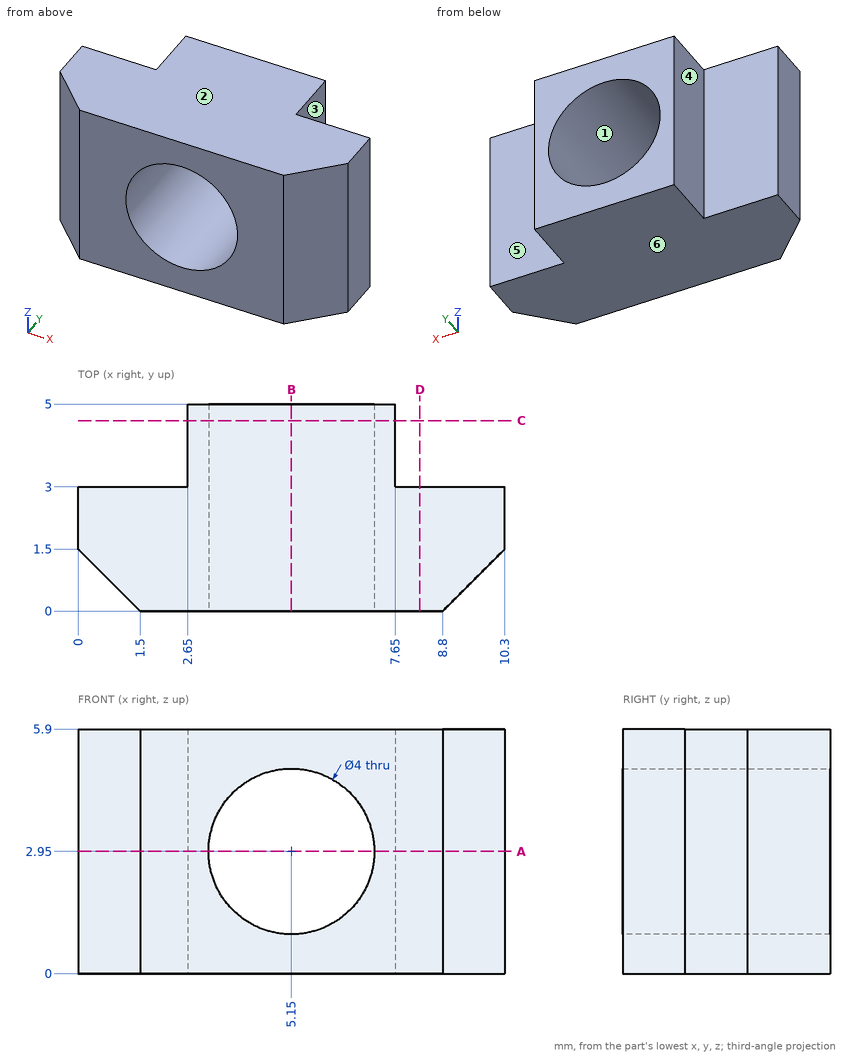
Source: three-view drawing plus pictorial views. Frame: mm from the lowest corner of the part. A direction names the side the tool comes from. Give positions to 0.01 mm unless a question says otherwise; leave off trailing zeros. Loops run counter-clockwise (first coordinate to the right, second up) from the corner with the lowest first, then second, coordinate; pieces in that order, holes last. Notation, with made-up numbers: M -16.75,12 L 3.25,12 A16 cw 3.25,22 Z; hole C 12,63 d1. An arc over 180 degrees is marked long. Use CSV: the item, a comma, the result in double quotes.
(1) Pull-direction query (X, two-part tool) for the marked faces 1, 2 and 3; classes: pulls with the +X half, pulls with the -X half, needs draft (parallel to the pull), parting line crosses it, or undercut.
Outcome:
face 1,"undercut"
face 2,"needs draft"
face 3,"pulls with the +X half"
(2) Set-up query: the marked faces 4, 5 and 6. Return all of +Z, -Z, +X, -X, +Y, -Y with unobstructed straight access to the full face (end or side cutting, diameter ignored); none if empty.
Outcome:
face 4,"+Z, -Z, -X, +Y"
face 5,"+Z, -Z, +X, +Y"
face 6,"-Z, +X, -X, +Y, -Y"
(3) Material intervals for L1, parallel to X at y = 3.75, z = 2.95; L2, parallel to X at y = 2, z = 2.95; L3, parallel to Y at x = 8.5, z = 4.3, sorted ascending. Write a range as [from, to].
Outcome:
L1,"x = [2.65, 3.15], [7.15, 7.65]"
L2,"x = [0, 3.15], [7.15, 10.3]"
L3,"y = [0, 3]"
(4) Section A-A, the plane z = 2.95. Return loops of the section in (x, y).
Outcome:
outline,"M 0,1.5 L 1.5,0 L 3.15,0 L 3.15,5 L 2.65,5 L 2.65,3 L 0,3 Z; M 7.15,0 L 8.8,0 L 10.3,1.5 L 10.3,3 L 7.65,3 L 7.65,5 L 7.15,5 Z"
(5) Pin query (flat end, axial travel): P1, Ø0.6, axis at y = 3.5, z = 3.5, coming from the -X side; P2, Ø1, axis at y = 4, z = 3, coming from the +X side. Return the tip coordinate at first contact, or that it passes through.
Outcome:
P1,"stops at x = 2.65"
P2,"stops at x = 7.65"
(6) Section D-D, the plane x = 8.25. Return loops of the section in (y, z), plus the area to 3 significant figures.
Outcome:
outline,"M 0,0 L 3,0 L 3,5.9 L 0,5.9 Z"
area,"17.7 mm²"
(7) Section B-B, the plane x = 5.15. Return loops of the section in (y, z), plus the area to 3 significant figures.
Outcome:
outline,"M 0,0 L 5,0 L 5,0.95 L 0,0.95 Z; M 0,4.95 L 5,4.95 L 5,5.9 L 0,5.9 Z"
area,"9.50 mm²"
(8) Section C-C, the plane y = 4.6. Return loops of the section in (x, z), plus the area to 3 significant figures.
Outcome:
outline,"M 2.65,0 L 7.65,0 L 7.65,5.9 L 2.65,5.9 Z; hole C 5.15,2.95 d4"
area,"16.9 mm²"
